For this review, take the finished solid that the model builds, in its own axes (mm). A direction names the side the tool comes from. Round coordinates to 2 decimals unless told otherwise and drop trailing zeros. Order: outer loops, then holes, each group sorted by start corner. A loop starts at its lowest first (then second) coordinate and runs counter-clockwise, first axis right, second up. Notation, with made-up numbers: (-18.75, 51.25) - (25.25, 51.25) arc R17 ccw to (25.25, 78.25) - close; hole circle Ø1 at (84, -27). An arc over 180 degrees is marked (long way). Write each question's results on one line, items separated by ' | '. Start each with the question number.
(1) Draft analysis for pull direction Y (two halves, no side actions). For faces 1 (the flat face through (-1, 1, 1.6)), 2 (the cylindrical face through (-13.77, -61.99, 0.79)), 3 (the cylindrical face through (44.41, -23.99, 0.79)), state which applies: pulls with the +Y half, pulls with the -Y half, needs draft (parallel to the pull), parting line crosses it, or undercut.
(2) Insertion check: pin 1 Ø0.8 at (x, z) = (-24.5, 0.5) entering from -Y; pin 2 Ø0.5 at (x, z) = (-54, 1) entering from -Y; pin 3 Ø0.8 at (x, z) = (52.5, 0.5) entering from +Y. Each pin has a flat end and moves straight along its axis. Give the tip position at first contact, or say it passes through.
(3) For L1, parallel to Y at x = 39, z = 1.1 (3 decimals); L2, parallel to X at y = -53, z = 0.8 (3 decimals); L3, parallel to X at y = 5, z = 0.75, list the stretches that pass through material, from the lowest coordinate up. Write a range as from..to.
(4) For faces 4 (the flat face through (-1, 1, 0)), 5 (the flat face through (33.118, 38.164, 0.789)), list the 3-axis set-ups (+Z, -Z, +X, -X, +Y, -Y) from which the entire face can be reached by the end or side of a thin tool; tool diameter is ignored.
(5) Take a section at D-D, the plane x = -30.5. Give the boundary of the cut face in (y, z), plus the area to 3 significant figures.
(6) Take a section at A-A, the plane y = 0. Give the boundary of the cut face in (x, z) (3 decimals), plus the area to 3 significant figures.
(7) Take a section at C-C, the plane z = 1.25. Give the number of separate pieces and of enclosed holes in the cut face, plus the area to 3 significant figures.
(8) Take a section at B-B, the plane y = 27. Give the boundary of the cut face in (x, z).
```python
from build123d import *

# Parameters (mm, degrees)
SKETCH1_R           = 63.5
BOSS_EXTRUDE1_DEPTH = 1.6
SKETCH3_R           = 1.75
CUT_EXTRUDE4_DEPTH  = 1.6
SKETCH2_R           = 1.5
CUT_EXTRUDE5_DEPTH  = 1.6
CUT_EXTRUDE6_DEPTH  = 10
SKETCH5_R           = 0.508001015
SKETCH5_W           = 3.45
SKETCH5_H           = 3.45
CUT_EXTRUDE7_DEPTH  = 10
SKETCH6_R           = 0.5
CUT_EXTRUDE8_DEPTH  = 10


with BuildPart() as part:
    # Sketch1 → Boss-Extrude1 (new body)
    with BuildSketch(Plane.XY):
        Circle(SKETCH1_R)
    extrude(amount=BOSS_EXTRUDE1_DEPTH)

    # Sketch3 → Cut-Extrude4 (cut)
    with BuildSketch(Plane(origin=(0, 0, 0), x_dir=(-1, 0, 0), z_dir=(0, 0, -1))):
        with Locations((-34.006305458, 36.654756705)):
            Circle(SKETCH3_R)
        with Locations((-49.354669589, 8.007283544)):
            Circle(SKETCH3_R)
    extrude(amount=-CUT_EXTRUDE4_DEPTH, mode=Mode.SUBTRACT)

    # Sketch2 → Cut-Extrude5 (cut)
    with BuildSketch(Plane(origin=(0, 0, 0), x_dir=(-1, 0, 0), z_dir=(0, 0, -1))):
        with Locations((0, 50)):
            Circle(SKETCH2_R)
        with Locations((43.301270189, -25)):
            Circle(SKETCH2_R)
        with Locations((-43.301270189, -25)):
            Circle(SKETCH2_R)
    extrude(amount=-CUT_EXTRUDE5_DEPTH, mode=Mode.SUBTRACT)

    # Sketch4 → Cut-Extrude6 (cut)
    with BuildSketch(Plane(origin=(0, 0, 0), x_dir=(-1, 0, 0), z_dir=(0, 0, -1))):
        with BuildLine():
            Line((-52.935522776, 11.911126581), (-44.12091565, 7.188553002))
            ThreePointArc((-44.12091565, 7.188553002), (-44.461118004, 5.385481223), (-45.773816402, 4.103440508))
            Line((-45.773816402, 4.103440508), (-54.588423529, 8.826014086))
            ThreePointArc((-54.588423529, 8.826014086), (-54.248221174, 10.629085865), (-52.935522776, 11.911126581))
        make_face()
        with BuildLine():
            Line((-39.240059397, 37.473487247), (-30.425452271, 32.750913668))
            ThreePointArc((-30.425452271, 32.750913668), (-29.112753873, 34.032954384), (-28.772551518, 35.836026163))
            Line((-28.772551518, 35.836026163), (-37.587158645, 40.558599742))
            ThreePointArc((-37.587158645, 40.558599742), (-38.899857043, 39.276559026), (-39.240059397, 37.473487247))
        make_face()
    extrude(amount=-CUT_EXTRUDE6_DEPTH, mode=Mode.SUBTRACT)

    # Sketch5 → Cut-Extrude7 (cut)
    with BuildSketch(Plane(origin=(0, 0, 0), x_dir=(-1, 0, 0), z_dir=(0, 0, -1))):
        with Locations((-10.219411384, -19.83547506)):
            Circle(SKETCH5_R)
        with Locations((-10.219411384, -22.37547506)):
            Circle(SKETCH5_R)
        with Locations((-10.219411384, -24.91547506)):
            Circle(SKETCH5_R)
        with Locations((-10.219411384, -27.45547506)):
            Circle(SKETCH5_R)
        with Locations((-10.219411384, -29.99547506)):
            Circle(SKETCH5_R)
        with Locations((-10.219411384, -32.53547506)):
            Circle(SKETCH5_R)
        with Locations((-10.219411384, -35.07547506)):
            Circle(SKETCH5_R)
        with Locations((-10.219411384, -37.61547506)):
            Circle(SKETCH5_R)
        with Locations((-10.219411384, -40.15547506)):
            Circle(SKETCH5_R)
        with Locations((-10.219411384, -42.69547506)):
            Circle(SKETCH5_R)
        with Locations((-10.219411384, -45.23547506)):
            Circle(SKETCH5_R)
        with Locations((-10.219411384, -47.77547506)):
            Circle(SKETCH5_R)
        with Locations((-10.219411384, -50.31547506)):
            Circle(SKETCH5_R)
        with Locations((-10.219411384, -52.85547506)):
            Circle(SKETCH5_R)
        with Locations((-10.219411384, -55.39547506)):
            Circle(SKETCH5_R)
        with Locations((-10.219411384, -57.93547506)):
            Circle(SKETCH5_R)
        with Locations((10.100588616, -57.93547506)):
            Circle(SKETCH5_R)
        with Locations((10.100588616, -55.39547506)):
            Circle(SKETCH5_R)
        with Locations((10.100588616, -52.85547506)):
            Circle(SKETCH5_R)
        with Locations((10.100588616, -50.31547506)):
            Circle(SKETCH5_R)
        with Locations((10.100588616, -47.77547506)):
            Circle(SKETCH5_R)
        with Locations((10.100588616, -45.23547506)):
            Circle(SKETCH5_R)
        with Locations((10.100588616, -42.69547506)):
            Circle(SKETCH5_R)
        with Locations((10.100588616, -40.15547506)):
            Circle(SKETCH5_R)
        with Locations((10.100588616, -37.61547506)):
            Circle(SKETCH5_R)
        with Locations((10.100588616, -29.99547506)):
            Circle(SKETCH5_R)
        with Locations((10.100588616, -32.53547506)):
            Circle(SKETCH5_R)
        with Locations((10.100588616, -35.07547506)):
            Circle(SKETCH5_R)
        Polygon((-14.856393822, 22.282028916), (-11.868606178, 24.007028916), (-10.143606178, 21.019241273), (-13.131393822, 19.294241273), align=None)
        with Locations((-25, 0)):
            Rectangle(SKETCH5_W, SKETCH5_H)
        with Locations((-40.24, 0)):
            Rectangle(SKETCH5_W, SKETCH5_H)
        with Locations((-52.94, 0)):
            Rectangle(SKETCH5_W, SKETCH5_H)
        Polygon((-22.476393822, 35.48025607), (-19.488606178, 37.20525607), (-17.763606178, 34.217468427), (-20.751393822, 32.492468427), align=None)
        Polygon((-28.826393822, 46.478778698), (-25.838606178, 48.203778698), (-24.113606178, 45.215991055), (-27.101393822, 43.490991055), align=None)
        Polygon((11.868606178, 24.007028916), (14.856393822, 22.282028916), (13.131393822, 19.294241273), (10.143606178, 21.019241273), align=None)
        Polygon((19.488606178, 37.20525607), (22.476393822, 35.48025607), (20.751393822, 32.492468427), (17.763606178, 34.217468427), align=None)
        Polygon((25.838606178, 48.203778698), (28.826393822, 46.478778698), (27.101393822, 43.490991055), (24.113606178, 45.215991055), align=None)
        with Locations((25, 0)):
            Rectangle(SKETCH5_W, SKETCH5_H)
        with Locations((40.24, 0)):
            Rectangle(SKETCH5_W, SKETCH5_H)
        with Locations((52.94, 0)):
            Rectangle(SKETCH5_W, SKETCH5_H)
        Polygon((22.476393822, -35.48025607), (19.488606178, -37.20525607), (17.763606178, -34.217468427), (20.751393822, -32.492468427), align=None)
        Polygon((28.826393822, -46.478778698), (25.838606178, -48.203778698), (24.113606178, -45.215991055), (27.101393822, -43.490991055), align=None)
        Polygon((-19.488606178, -37.20525607), (-22.476393822, -35.48025607), (-20.751393822, -32.492468427), (-17.763606178, -34.217468427), align=None)
        Polygon((-25.838606178, -48.203778698), (-28.826393822, -46.478778698), (-27.101393822, -43.490991055), (-24.113606178, -45.215991055), align=None)
    extrude(amount=-CUT_EXTRUDE7_DEPTH, mode=Mode.SUBTRACT)

    # Sketch6 → Cut-Extrude8 (cut)
    with BuildSketch(Plane(origin=(0, 0, 0), x_dir=(-1, 0, 0), z_dir=(0, 0, -1))):
        with Locations((0, 4.75)):
            Circle(SKETCH6_R)
        with Locations((-3.358757211, 3.358757211)):
            Circle(SKETCH6_R)
        with Locations((3.358757211, 3.358757211)):
            Circle(SKETCH6_R)
        with Locations(Location((3.358757211, -3.358757211, 0), (0, 0, 180))):
            Circle(SKETCH6_R)
        with Locations(Location((0, -4.75, 0), (0, 0, 180))):
            Circle(SKETCH6_R)
        with Locations(Location((-3.358757211, -3.358757211, 0), (0, 0, 180))):
            Circle(SKETCH6_R)
    extrude(amount=-CUT_EXTRUDE8_DEPTH, mode=Mode.SUBTRACT)


solid = part.part
```
Results below:
1) face 1: needs draft | face 2: parting line crosses it | face 3: undercut
2) pin 1: stops at y = -58.75 | pin 2: stops at y = -33.81 | pin 3: stops at y = 36.3
3) L1: y = -50.112..-1.725, 1.725..37.345, 39.072..50.112 | L2: x = -34.975..-10.588, -9.614..9.732, 10.706..34.975 | L3: x = -63.3..-0.43, 0.43..44.71, 47.45..63.3
4) face 4: -Z, +X, -X, +Y, -Y | face 5: +Z, -Z
5) outline: (-55.7, 0) - (55.7, 0) - (55.7, 1.6) - (-55.7, 1.6) - close | area: 178 mm^2
6) outline: (-63.5, 0) - (-54.665, 0) - (-54.665, 1.6) - (-63.5, 1.6) - close; (-51.215, 0) - (-41.965, 0) - (-41.965, 1.6) - (-51.215, 1.6) - close; (-38.515, 0) - (-26.725, 0) - (-26.725, 1.6) - (-38.515, 1.6) - close; (-23.275, 0) - (23.275, 0) - (23.275, 1.6) - (-23.275, 1.6) - close; (26.725, 0) - (38.515, 0) - (38.515, 1.6) - (26.725, 1.6) - close; (41.965, 0) - (51.215, 0) - (51.215, 1.6) - (41.965, 1.6) - close; (54.665, 0) - (63.5, 0) - (63.5, 1.6) - (54.665, 1.6) - close | area: 170 mm^2
7) separate pieces: 1 | enclosed holes: 55 | area: 12,400 mm^2
8) outline: (-57.47, 0) - (57.47, 0) - (57.47, 1.6) - (-57.47, 1.6) - close
